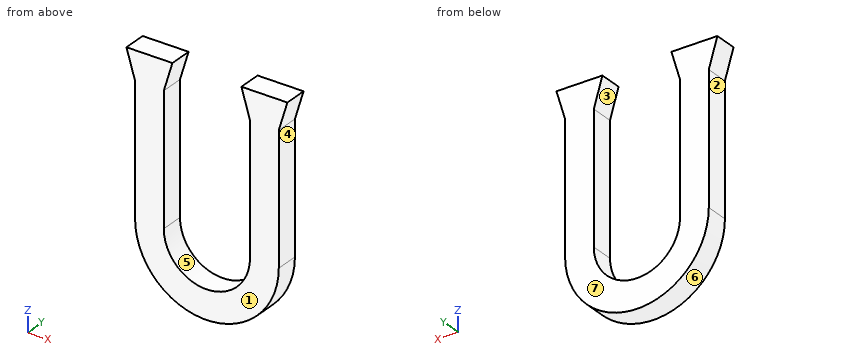
from build123d import *

# Parameters (mm, degrees)
F1_DEPTH = 5.08


with BuildPart() as f1:
    # F0 (on Front) → F1 (new body)
    with BuildSketch(Plane.XZ):
        with BuildLine():
            Line((-15.875, 28.575), (-15.875, 0))
            ThreePointArc((-15.875, 0), (0, -15.875), (15.875, 0))
            Line((15.875, 0), (15.875, 28.575))
            Line((15.875, 28.575), (17.78, 34.925))
            Line((17.78, 34.925), (15.875, 34.925))
            Line((15.875, 34.925), (9.525, 34.925))
            Line((9.525, 34.925), (7.62, 34.925))
            Line((7.62, 34.925), (9.525, 28.575))
            Line((9.525, 28.575), (9.525, 0))
            ThreePointArc((9.525, 0), (0, -9.525), (-9.525, 0))
            Line((-9.525, 0), (-9.525, 28.575))
            Line((-9.525, 28.575), (-7.62, 34.925))
            Line((-7.62, 34.925), (-9.525, 34.925))
            Line((-9.525, 34.925), (-15.875, 34.925))
            Line((-15.875, 34.925), (-17.78, 34.925))
            Line((-17.78, 34.925), (-15.875, 28.575))
        make_face()
    extrude(amount=F1_DEPTH)


solid = f1.part
Source: CAD feature listing. Evaluate the final solid. Frame: model axes, mm. Face numbers are marked on the shaded views. A direction names the side the tool comes from. Round coordinates to 2 decimals unless told otherwise and drop trailing zeros. Order: outer loops, then holes, each group sorted by start corner. A loop starts at its lowest first (then second) coordinate and runs counter-clockwise, first axis right, second up. Notation, with made-up numbers: (-29.5, -38.75) - (17.5, -38.75) arc R33 cw to (17.5, -8.75) - close; hole circle Ø4 at (45.25, 15). An arc over 180 degrees is marked (long way). Use a Markdown table: item, result. Add a question column.
1. Line query: probe 1 along X at (y, z) = (-1.8, 2.5) (3 decimals); probe 2 along X at (y, z) = (-4.2, -2); probe 3 along Z at (x, y) = (0, -2.25) (3 decimals). Output: solid intervals per line, ascending.
2. Mould query, pull axis X, two halves, no side actions, for the marked faces 5, 6 and 7. Classes: +X half, -X half, draft (parallel to the pull), parting line (faces both ways), or undercut.
3. First-contact query: pin 1 (1 mm diameter, centred on y = -4, z = 8, fed in from +X) (3 decimals); pin 2 (3 mm diameter, centred on x = -4.5, y = -4.5, fed in from +Z); pin 3 (3 mm diameter, centred on x = -2.5, y = -4, fed in from +Z); pin 4 (12 mm diameter, centred on x = 1, z = 13, fed in from +Y). Flat tips, straight axial feed; report the tip coordinate or a pass-through.
4. Section query A-A (z = 2). Return the cut outline in (x, y) (3 decimals), then the cut area to 3 significant figures.
5. Section query C-C (x = 0). Return the cut outline in (y, z) (3 decimals), then the cut area to 3 significant figures.
6. Section query D-D (z = 30). Return the cut outline in (x, y), then the cut area to 3 significant figures.
7. Section query B-B (y = -4.1). Return the cut outline in (x, z) (3 decimals).
8. Set-up query: the marked faces 1, 2, 3 and 4. Return all of +Z, -Z, +X, -X, +Y, -Y with unobstructed straight access to the full face (end or side cutting, diameter ignored); none if empty.
Derived:
| question | item | result |
|---|---|---|
| 1 | probe 1 | -15.875 to -9.525, 9.525 to 15.875 |
| 1 | probe 2 | -15.75 to -9.31, 9.31 to 15.75 |
| 1 | probe 3 | -15.875 to -9.525 |
| 2 | face 5 | undercut |
| 2 | face 6 | parting line |
| 2 | face 7 | draft |
| 3 | pin 1 | x = 15.875 |
| 3 | pin 2 | z = -7.4 |
| 3 | pin 3 | z = -8.64 |
| 3 | pin 4 | through |
| 4 | outline | (-15.875, -5.08) - (-9.525, -5.08) - (-9.525, 0) - (-15.875, 0) - close; (9.525, -5.08) - (15.875, -5.08) - (15.875, 0) - (9.525, 0) - close |
| 4 | area | 64.5 mm2 |
| 5 | outline | (-5.08, -15.875) - (0, -15.875) - (0, -9.525) - (-5.08, -9.525) - close |
| 5 | area | 32.3 mm2 |
| 6 | outline | (-16.3, -5.08) - (-9.1, -5.08) - (-9.1, 0) - (-16.3, 0) - close; (9.1, -5.08) - (16.3, -5.08) - (16.3, 0) - (9.1, 0) - close |
| 6 | area | 73.2 mm2 |
| 7 | outline | (-17.78, 34.925) - (-15.875, 28.575) - (-15.875, 0) arc R15.875 ccw to (15.875, 0) - (15.875, 28.575) - (17.78, 34.925) - (7.62, 34.925) - (9.525, 28.575) - (9.525, 0) arc R9.525 cw to (-9.525, 0) - (-9.525, 28.575) - (-7.62, 34.925) - close |
| 8 | face 1 | +Z, -Z, +X, -X, -Y |
| 8 | face 2 | -Z, -X, +Y, -Y |
| 8 | face 3 | +Y, -Y |
| 8 | face 4 | -Z, +X, +Y, -Y |
